Here's how the part is built. I have some questions about the finished solid (model axes, mm). A direction names the side the tool comes from. Coordinates: 2 decimals unless noted, no trailing zeros. Loops run counter-clockwise (first coordinate to the right, second up) from the corner with the lowest first, then second, coordinate; pieces in that order, holes last. Notation, with made-up numbers: (30, 29) - (40, 29) arc R21 ccw to (40, 47) - close; hole circle Ø11 at (-7.75, 10). An arc over 180 degrees is marked (long way). Use a Markdown table: item, result.
```python
from build123d import *

# Parameters (mm, degrees)
SKETCH1_R           = 1.5
SKETCH1_W           = 3.45
SKETCH1_H           = 15
SKETCH1_W_2         = 30
SKETCH1_H_2         = 3.45
BOSS_EXTRUDE1_DEPTH = 3.3


with BuildPart() as part:
    # Sketch1 → Boss-Extrude1 (new body)
    with BuildSketch(Plane(origin=(0, 0, 0), x_dir=(1, 0, 0), z_dir=(0, 1, 0))):
        with BuildLine():
            Line((-35, 35), (35, 35))
            ThreePointArc((35, 35), (42.071067812, 32.071067812), (45, 25))
            Line((45, 25), (45, -25))
            ThreePointArc((45, -25), (42.071067812, -32.071067812), (35, -35))
            Line((35, -35), (-35, -35))
            ThreePointArc((-35, -35), (-42.071067812, -32.071067812), (-45, -25))
            Line((-45, -25), (-45, 25))
            ThreePointArc((-45, 25), (-42.071067812, 32.071067812), (-35, 35))
        make_face()
        with Locations(Location((-35, -25, 0), (0, 0, 270))):
            Circle(SKETCH1_R, mode=Mode.SUBTRACT)
        with Locations(Location((-35, -15, 0), (0, 0, 270))):
            Circle(SKETCH1_R, mode=Mode.SUBTRACT)
        with Locations(Location((-35, -5, 0), (0, 0, 270))):
            Circle(SKETCH1_R, mode=Mode.SUBTRACT)
        with Locations(Location((-35, 5, 0), (0, 0, 270))):
            Circle(SKETCH1_R, mode=Mode.SUBTRACT)
        with Locations(Location((-35, 15, 0), (0, 0, 270))):
            Circle(SKETCH1_R, mode=Mode.SUBTRACT)
        with Locations(Location((-35, 25, 0), (0, 0, 270))):
            Circle(SKETCH1_R, mode=Mode.SUBTRACT)
        with Locations(Location((-25, -25, 0), (0, 0, 270))):
            Circle(SKETCH1_R, mode=Mode.SUBTRACT)
        with Locations(Location((-25, -15, 0), (0, 0, 270))):
            Circle(SKETCH1_R, mode=Mode.SUBTRACT)
        with Locations(Location((-25, -5, 0), (0, 0, 270))):
            Circle(SKETCH1_R, mode=Mode.SUBTRACT)
        with Locations(Location((-25, 5, 0), (0, 0, 270))):
            Circle(SKETCH1_R, mode=Mode.SUBTRACT)
        with Locations(Location((-25, 15, 0), (0, 0, 270))):
            Circle(SKETCH1_R, mode=Mode.SUBTRACT)
        with Locations(Location((-25, 25, 0), (0, 0, 270))):
            Circle(SKETCH1_R, mode=Mode.SUBTRACT)
        with Locations(Location((-15, -15, 0), (0, 0, 270))):
            Circle(SKETCH1_R, mode=Mode.SUBTRACT)
        with Locations(Location((-15, -5, 0), (0, 0, 270))):
            Circle(SKETCH1_R, mode=Mode.SUBTRACT)
        with Locations(Location((-15, 5, 0), (0, 0, 270))):
            Circle(SKETCH1_R, mode=Mode.SUBTRACT)
        with Locations(Location((-15, 15, 0), (0, 0, 270))):
            Circle(SKETCH1_R, mode=Mode.SUBTRACT)
        with Locations(Location((-15, 25, 0), (0, 0, 270))):
            Circle(SKETCH1_R, mode=Mode.SUBTRACT)
        with Locations(Location((15, -15, 0), (0, 0, 270))):
            Circle(SKETCH1_R, mode=Mode.SUBTRACT)
        with Locations(Location((15, -5, 0), (0, 0, 270))):
            Circle(SKETCH1_R, mode=Mode.SUBTRACT)
        with Locations(Location((15, 5, 0), (0, 0, 270))):
            Circle(SKETCH1_R, mode=Mode.SUBTRACT)
        with Locations(Location((15, 15, 0), (0, 0, 270))):
            Circle(SKETCH1_R, mode=Mode.SUBTRACT)
        with Locations(Location((15, 25, 0), (0, 0, 270))):
            Circle(SKETCH1_R, mode=Mode.SUBTRACT)
        with Locations(Location((25, -25, 0), (0, 0, 270))):
            Circle(SKETCH1_R, mode=Mode.SUBTRACT)
        with Locations(Location((25, -15, 0), (0, 0, 270))):
            Circle(SKETCH1_R, mode=Mode.SUBTRACT)
        with Locations(Location((25, -5, 0), (0, 0, 270))):
            Circle(SKETCH1_R, mode=Mode.SUBTRACT)
        with Locations(Location((25, 5, 0), (0, 0, 270))):
            Circle(SKETCH1_R, mode=Mode.SUBTRACT)
        with Locations(Location((25, 15, 0), (0, 0, 270))):
            Circle(SKETCH1_R, mode=Mode.SUBTRACT)
        with Locations(Location((25, 25, 0), (0, 0, 270))):
            Circle(SKETCH1_R, mode=Mode.SUBTRACT)
        with Locations(Location((35, -25, 0), (0, 0, 270))):
            Circle(SKETCH1_R, mode=Mode.SUBTRACT)
        with Locations(Location((35, -15, 0), (0, 0, 270))):
            Circle(SKETCH1_R, mode=Mode.SUBTRACT)
        with Locations(Location((35, -5, 0), (0, 0, 270))):
            Circle(SKETCH1_R, mode=Mode.SUBTRACT)
        with Locations(Location((35, 5, 0), (0, 0, 270))):
            Circle(SKETCH1_R, mode=Mode.SUBTRACT)
        with Locations(Location((35, 15, 0), (0, 0, 270))):
            Circle(SKETCH1_R, mode=Mode.SUBTRACT)
        with Locations(Location((35, 25, 0), (0, 0, 270))):
            Circle(SKETCH1_R, mode=Mode.SUBTRACT)
        with Locations((0, -7.5)):
            Rectangle(SKETCH1_W, SKETCH1_H, mode=Mode.SUBTRACT)
        with Locations((0, 17.5)):
            Rectangle(SKETCH1_W, SKETCH1_H, mode=Mode.SUBTRACT)
        with Locations((0, -26.725)):
            Rectangle(SKETCH1_W_2, SKETCH1_H_2, mode=Mode.SUBTRACT)
    extrude(amount=BOSS_EXTRUDE1_DEPTH)


solid = part.part
```
Q1. Which directions (+Z, -Z, +X, -X, +Y, -Y) give clear straight access to the entire face, cutting with the end or side of a thin tool? Please do faces 1 (the face through (-1.725, 2, 8)), 2 (the face through (-45, 2, 0)).
Check values:
| item | result |
|---|---|
| face 1 | +Y, -Y |
| face 2 | +Z, -Z, -X, +Y, -Y |
Q2. Will this pin go through, and if not, where does the flat tip stop? P1, Ø2.5, axis at x = -25, z = 15, coming from the +Y side.
Check values:
| item | result |
|---|---|
| P1 | through |
Q3. I want a section at D-D, the plane z = 5. Give the number of separate pieces and of enclosed holes in the cut face, then the cut area to 3 significant figures.
Check values:
| item | result |
|---|---|
| separate pieces | 8 |
| enclosed holes | 0 |
| area | 226 mm^2 |
Q4. I want a section at B-B, the plane z = -11.5. Write out the boundary of the cut face in (x, y) (3 decimals).
Check values:
| item | result |
|---|---|
| outline | (-45, 0) - (-1.725, 0) - (-1.725, 3.3) - (-45, 3.3) - close; (1.725, 0) - (45, 0) - (45, 3.3) - (1.725, 3.3) - close |
Q5. Please list where these lines run through material, in increasing order: L1, parallel to Z at x = -2, y = 2.55; L2, parallel to X at y = 2, z = 7 (3 decimals); L3, parallel to X at y = 1.7, z = 24. Write a range as from..to.
Check values:
| item | result |
|---|---|
| L1 | -35..25, 28.45..35 |
| L2 | -45..-1.725, 1.725..45 |
| L3 | -45..-36.12, -33.88..-26.12, -23.88..23.88, 26.12..33.88, 36.12..45 |
Q6. I want a section at C-C, the plane x = 5. Write out the boundary of the cut face in (y, z).
Check values:
| item | result |
|---|---|
| outline | (0, -35) - (3.3, -35) - (3.3, 25) - (0, 25) - close; (0, 28.45) - (3.3, 28.45) - (3.3, 35) - (0, 35) - close |
Q7. I want a section at A-A, the plane x = 25. Write out the boundary of the cut face in (y, z), then the cut area to 3 significant figures.
Check values:
| item | result |
|---|---|
| outline | (0, -35) - (3.3, -35) - (3.3, -26.5) - (0, -26.5) - close; (0, -23.5) - (3.3, -23.5) - (3.3, -16.5) - (0, -16.5) - close; (0, -13.5) - (3.3, -13.5) - (3.3, -6.5) - (0, -6.5) - close; (0, -3.5) - (3.3, -3.5) - (3.3, 3.5) - (0, 3.5) - close; (0, 6.5) - (3.3, 6.5) - (3.3, 13.5) - (0, 13.5) - close; (0, 16.5) - (3.3, 16.5) - (3.3, 23.5) - (0, 23.5) - close; (0, 26.5) - (3.3, 26.5) - (3.3, 35) - (0, 35) - close |
| area | 172 mm^2 |
Q8. If we mould it in two halves opening along X, with no side actions, what happens to faces 3 (the face through (26.01, 1.63, -26.11)), 4 (the face through (-41.99, 1.63, 32.15)), 5 (the face through (-36.464, 1.627, 4.675)), 6 (the face through (0.6, 0, -0.5))? For each: pulls with the +X half, pulls with the -X half, needs draft (parallel to the pull), parting line crosses it, or undercut.
Check values:
| item | result |
|---|---|
| face 3 | undercut |
| face 4 | pulls with the -X half |
| face 5 | undercut |
| face 6 | needs draft |
